Verification items for the finished model (mm, model axes). A direction names the side the tool comes from. Give positions to 0.01 mm unless a question says otherwise; leave off trailing zeros. Loops run counter-clockwise (first coordinate to the right, second up) from the corner with the lowest first, then second, coordinate; pieces in that order, holes last. Notation, with made-up numbers: M 61.25,-3.75 L 67.25,-3.75 A16 cw 67.25,15.25 Z; hole C 70,-20 d11. An arc over 180 degrees is marked long. Use CSV: the item, a comma, the result in double quotes.
from build123d import *

# Parameters (mm, degrees)
SKETCH1_R                = 3
BOSS_EXTRUDE1_DEPTH      = 25.68
REVOLVE1_ANGLE           = 100
REVOLVE1_OTHER_WAY_ANGLE = 100
BOSS_EXTRUDE2_DEPTH      = 20


with BuildPart() as part:
    # Sketch1 → Boss-Extrude1 (new body)
    with BuildSketch(Plane(origin=(0, 0, 0), x_dir=(1, 0, 0), z_dir=(0, 1, 0))):
        with Locations(Location((0, 0, 0), (0, 0, 90))):
            Circle(SKETCH1_R)
    extrude(amount=BOSS_EXTRUDE1_DEPTH)

    # Sketch3 → Revolve1 (revolve)
    with BuildSketch(Plane(origin=(0, 0, 0), x_dir=(0, 0, -1), z_dir=(1, 0, 0))):
        Polygon((1, 31.68), (5, 25.68), (0, 25.68), (0, 31.68), align=None)
    revolve(axis=Axis((0, 25.68, 0), (0, 1, 0)), revolution_arc=REVOLVE1_ANGLE)

    # Sketch3 → Revolve1 other way (revolve)
    with BuildSketch(Plane(origin=(0, 0, 0), x_dir=(0, 0, -1), z_dir=(1, 0, 0))):
        Polygon((1, 31.68), (5, 25.68), (0, 25.68), (0, 31.68), align=None)
    revolve(axis=Axis((0, 25.68, 0), (0, -1, 0)), revolution_arc=REVOLVE1_OTHER_WAY_ANGLE)

    # Sketch4 → Boss-Extrude2 (add)
    with BuildSketch(Plane(origin=(0, 0, 0), x_dir=(-1, 0, 0), z_dir=(0, -1, 0))):
        with BuildLine():
            ThreePointArc((2.833333333, -0.986013297), (2.999990846, 0.007411119), (2.828427125, 1))
            Line((2.828427125, 1), (3.833333333, 1))
            Line((3.833333333, 1), (3.833333333, -0.986013297))
            Line((3.833333333, -0.986013297), (2.833333333, -0.986013297))
        make_face()
        with BuildLine():
            Line((-3.833333333, -0.986013297), (-2.833333333, -0.986013297))
            ThreePointArc((-2.833333333, -0.986013297), (-2.999990846, 0.007411119), (-2.828427125, 1))
            Line((-2.828427125, 1), (-3.833333333, 1))
            Line((-3.833333333, 1), (-3.833333333, -0.986013297))
        make_face()
    extrude(amount=-BOSS_EXTRUDE2_DEPTH)


solid = part.part
(1) Mould release check, pull along Y, two halves, no side actions. Record for faces 1 (the conical face through (-0.063, 29.305, -2.583)), 2 (the flat face through (0, 0, 0)), 3 (the flat face through (-3, 10, 0.986)), 4 (the flat face through (-3.3, 20, 0)): released by +Y, released by -Y, zero draft, split by the parting line, or undercut.
Calculated:
face 1,"released by +Y"
face 2,"released by -Y"
face 3,"zero draft"
face 4,"undercut"
(2) Section check B-B on z = 1.5. Record the cut outline in (x, y), plus the area to 3 significant figures.
Calculated:
outline,"M -2.6,0 L 2.6,0 L 2.6,25.68 L -2.6,25.68 Z"
area,"133 mm²"
(3) Depth check by flat-ended pin: pin 1 Ø1.5 at (x, z) = (1, 1.5) entering from +Y; pin 2 Ø1.1 at (x, y) = (3.5, 5) entering from -Z; pin 3 Ø1 at (y, z) = (7, 0) entering from +X. Enter the tip coordinate at first touch or a pass-through.
Calculated:
pin 1,"stops at y = 25.68"
pin 2,"stops at z = -1"
pin 3,"stops at x = 3.83"
(4) Scan lines: L1, parallel to Z at x = 3.5, y = 2; L2, parallel to Y at x = 1.25, z = 2.5; L3, parallel to X at y = 4, z = -0.5. Record each from-to range of solid material in increasing order. Write a range as from..to.
Calculated:
L1,"z = -1..0.99"
L2,"y = 0..25.68"
L3,"x = -3.83..3.83"
(5) Tool access check on faces 5 (the flat face through (3, 10, -1)), 6 (the flat face through (0, 25.68, 2)), 7 (the flat face through (3, 10, 0.986)), 8 (the flat face through (0.1, 25.68, -3.3)), 9 (the flat face through (3.833, 10, 0)). Record the directions out of +Z, -Z, +X, -X, +Y, -Y that give a thin tool (end or side, any length) a straight path to the whole face; none if there is none.
Calculated:
face 5,"-Z, +X, -Y"
face 6,"+Z, +Y"
face 7,"+Z, +X, +Y, -Y"
face 8,"-Z"
face 9,"+Z, -Z, +X, -Y"
(6) Section check A-A on y = 12.5. Record the cut outline in (x, z), plus the area to 3 significant figures.
Calculated:
outline,"M -3.83,-1 L -2.83,-1 A3 ccw 2.83,-1 L 3.83,-1 L 3.83,0.99 L 2.83,0.99 A3 ccw -2.83,0.99 L -3.83,0.99 Z"
area,"31.8 mm²"
